Verification items for the finished model (mm, model axes). A direction names the side the tool comes from. Round coordinates to 2 decimals unless told otherwise and drop trailing zeros. Order: outer loops, then holes, each group sorted by start corner. A loop starts at its lowest first (then second) coordinate and runs counter-clockwise, first axis right, second up. Notation, with made-up numbers: (64.25, 51.25) -> (83.25, 51.25) arc R27 cw to (83.25, 90.25) -> close; hole circle Ø8 at (16.5, 13). An arc over 180 degrees is marked (long way). Answer in a Markdown table with one row per item. Add a question column.
```python
from build123d import *

# Parameters (mm, degrees)
SKETCH1_W          = 426.72
SKETCH1_H          = 5
EXTRUDE2_DEPTH     = 16
SKETCH2_R          = 5
EXTRUDE3_DEPTH     = 5
SKETCH3_W          = 6
SKETCH3_H          = 40.995425817
CUT_EXTRUDE1_DEPTH = 13.626819
SKETCH4_R          = 5
EXTRUDE4_DEPTH     = 3.5


with BuildPart() as part:
    # Sketch1 → Extrude2 (new body, symmetric)
    with BuildSketch(Plane(origin=(0, 0, 0), x_dir=(1, 0, 0), z_dir=(0, 0, -1))):
        with Locations((213.36, 0)):
            Rectangle(SKETCH1_W, SKETCH1_H)
    extrude(amount=EXTRUDE2_DEPTH, both=True)

    # Sketch2 → Extrude3 (add, symmetric)
    with BuildSketch(Plane.XY):
        with BuildLine():
            Line((0.803073324, 2.5), (0.803073324, 16.921503506))
            ThreePointArc((0.803073324, 16.921503506), (7.616482736, 23.734912918), (14.429892147, 16.921503506))
            Line((14.429892147, 16.921503506), (14.429892147, 2.5))
            Line((14.429892147, 2.5), (0.803073324, 2.5))
        make_face()
        with Locations((7.616482736, 16.921503506)):
            Circle(SKETCH2_R, mode=Mode.SUBTRACT)
    extrude(amount=EXTRUDE3_DEPTH, both=True)

    # Sketch3 → Cut-Extrude1 (cut)
    with BuildSketch(Plane.ZY.offset(-0.803073324)):
        with Locations((0, 22.997712909)):
            Rectangle(SKETCH3_W, SKETCH3_H)
    extrude(amount=-CUT_EXTRUDE1_DEPTH, mode=Mode.SUBTRACT)

    # Sketch4 → Extrude4 (add, symmetric)
    with BuildSketch(Plane.XY):
        with BuildLine():
            Line((408.398633308, 2.5), (408.398633308, 18.51574669))
            ThreePointArc((408.398633308, 18.51574669), (397.805657025, 29.108722972), (387.212680742, 18.51574669))
            Line((387.212680742, 18.51574669), (387.212680742, 2.5))
            Line((387.212680742, 2.5), (408.398633308, 2.5))
        make_face()
        with Locations((397.805657025, 18.51574669)):
            Circle(SKETCH4_R, mode=Mode.SUBTRACT)
    extrude(amount=EXTRUDE4_DEPTH, both=True)


solid = part.part
```
1) Tool access check on faces 4 (the face through (8, 11, 3)), 5 (the face through (8, 11, 5)), 6 (the face through (398, 13, -3.5)), 7 (the face through (8, 11, -5)), 8 (the face through (387.213, 11, 0)). Record the directions out of +Z, -Z, +X, -X, +Y, -Y that give a thin tool (end or side, any length) a straight path to the whole face; none if there is none.
2) Cross-section at A-A, the plane y = 7.5. Record the boundary of the cut face in (x, z).
3) Depth check by flat-ended pin: P1, Ø1, axis at y = 11.5, z = -4, coming from the -X side; P2, Ø8, axis at x = 303.5, z = -8.5, coming from the +Y side; P3, Ø0.6, axis at y = 11.5, z = 4, coming from the +X side. Enter the tip coordinate at first touch or a pass-through.
4) Cross-section at B-B, the plane x = 54. Record the boundary of the cut face in (y, z).
5) Thickness scan on L1, parallel to Y at x = 114, z = -3.5; L2, parallel to X at y = 8, z = 0.5. Record the ranges inside material, lowest first. Write a range as [from, to].
6) Draft check along X on faces 1 (the face through (3.93, 20.3, 3.99)), 2 (the face through (398, 13, 3.5)), 3 (the face through (408.399, 10, 0)). Enter one of: +X half, -X half, draft (parallel to the pull), parting line (faces both ways), or undercut.
Results below:
| question | item | result |
|---|---|---|
| 1 | face 4 | -X, +Y |
| 1 | face 5 | +Z, +X, -X, +Y |
| 1 | face 6 | -Z, +X, +Y |
| 1 | face 7 | -Z, +X, -X, +Y |
| 1 | face 8 | +Z, -Z, +Y |
| 2 | outline | (0.8, -5) -> (14.43, -5) -> (14.43, -3) -> (0.8, -3) -> close; (0.8, 3) -> (14.43, 3) -> (14.43, 5) -> (0.8, 5) -> close; (387.21, -3.5) -> (408.4, -3.5) -> (408.4, 3.5) -> (387.21, 3.5) -> close |
| 3 | P1 | x = 0.8 |
| 3 | P2 | y = 2.5 |
| 3 | P3 | x = 14.43 |
| 4 | outline | (-2.5, -16) -> (2.5, -16) -> (2.5, 16) -> (-2.5, 16) -> close |
| 5 | L1 | [-2.5, 2.5] |
| 5 | L2 | [387.21, 408.4] |
| 6 | face 1 | undercut |
| 6 | face 2 | draft |
| 6 | face 3 | +X half |
